```python
from build123d import *

# Parameters (mm, degrees)
F0_W      = 38
F0_H      = 28.5
F1_DEPTH  = 19.5
F2_W      = 8
F2_H      = 15.5
F4_DEPTH  = 38
F6_DEPTH  = 19.5
F3_W      = 10
F3_H      = 9
F7_DEPTH  = 38
F9_DEPTH  = 38
F11_DEPTH = 7
F12_W     = 32
F12_H     = 5
F13_DEPTH = 19
F14_R     = 2
F15_DEPTH = 4


with BuildPart() as f1:
    # F0 (on Top) → F1 (new body)
    with BuildSketch(Plane.XY):
        with Locations((3.113019, 14.25)):
            Rectangle(F0_W, F0_H)
    extrude(amount=F1_DEPTH)

    # F2 (on face) → F4 (cut)
    with BuildSketch(Plane.YZ.offset(22.113019)):
        with Locations((4, 11.75)):
            Rectangle(F2_W, F2_H)
    extrude(amount=-F4_DEPTH, mode=Mode.SUBTRACT)

    # F5 (on face) → F6 (cut)
    with BuildSketch(Plane.XY.offset(19.5)):
        with BuildLine():
            ThreePointArc((-8.449312, 27.5), (-11.386981, 18.75), (-8.449312, 10))
            Line((-8.449312, 10), (14.67535, 10))
            ThreePointArc((14.67535, 10), (17.613019, 18.75), (14.67535, 27.5))
            Line((14.67535, 27.5), (-8.449312, 27.5))
        make_face()
    extrude(amount=-F6_DEPTH, mode=Mode.SUBTRACT)

    # F3 (on face) → F7 (cut)
    with BuildSketch(Plane.YZ.offset(22.113019)):
        with Locations((23.5, 15)):
            Rectangle(F3_W, F3_H)
    extrude(amount=-F7_DEPTH, mode=Mode.SUBTRACT)

    # F8 (on face) → F9 (cut)
    with BuildSketch(Plane.YZ.offset(22.113019)):
        Polygon((18.5, 19.5), (8, 19.5), (8, 14), (10.5, 11.5), align=None)
    extrude(amount=-F9_DEPTH, mode=Mode.SUBTRACT)

    # F10 (on face) → F11 (cut)
    with BuildSketch(Plane(origin=(0, 0, 0), x_dir=(1, 0, 0), z_dir=(0, 0, -1))):
        with BuildLine():
            Line((15.550362, -9.5), (-9.324324, -9.5))
            ThreePointArc((-9.324324, -9.5), (-12.386981, -18.75), (-9.324324, -28))
            Line((-9.324324, -28), (15.550362, -28))
            ThreePointArc((15.550362, -28), (18.613019, -18.75), (15.550362, -9.5))
        make_face()
    extrude(amount=-F11_DEPTH, mode=Mode.SUBTRACT)

    # F12 (on face) → F13 (cut)
    with BuildSketch(Plane(origin=(0, 28.5, 0), x_dir=(-1, 0, 0), z_dir=(0, 1, 0))):
        with Locations((-3.113019, 2.5)):
            Rectangle(F12_W, F12_H)
    extrude(amount=-F13_DEPTH, mode=Mode.SUBTRACT)

    # F14 (on face) → F15 (cut)
    with BuildSketch(Plane.XY.offset(4)):
        with Locations((-5.136981, 4.25)):
            Circle(F14_R)
        with Locations((11.363019, 4.25)):
            Circle(F14_R)
    extrude(amount=-F15_DEPTH, mode=Mode.SUBTRACT)


solid = f1.part
```
Verification items for the finished model (mm, model axes). A direction names the side the tool comes from. Round coordinates to 2 decimals unless told otherwise and drop trailing zeros. Write each loop counter-clockwise with the first axis right and the second up, starting at its lowest first coordinate (ties: lowest second). Pieces come first, ordered by that corner, then holes. Notation, with made-up numbers: (31, -29) - (90, -29) arc R22 cw to (90, -18) - close; hole circle Ø2 at (20.5, -10). An arc over 180 degrees is marked (long way). Answer as a JSON object with one key per item and string values. Group by question number.
Q1. Tool access check on faces 1 (the flat face through (-13, 14, 15)), 2 (the flat face through (20, 18.5, 15)), 3 (the flat face through (3, 9.5, 4)). Record the directions out of +Z, -Z, +X, -X, +Y, -Y that give a thin tool (end or side, any length) a straight path to the whole face; none if there is none.
Q2. Go/stop test with flat-tipped pins: pin 1 Ø1.4 at (x, z) = (-13.5, 15) entering from +Y; pin 2 Ø1 at (x, z) = (9, 6.5) entering from -Y; pin 3 Ø4 at (x, y) = (-5, 3.5) entering from +Z; pin 4 Ø7.5 at (x, z) = (-1.5, 3.5) entering from +Y. Record where each tip stops, or that it passes through.
Q3. Section check C-C, the plane x = 7. Enter the section's corners in (y, z), plus the area to 3 significant figures.
Q4. Section check B-B, the plane z = 7.5. Enter the section's corners in (x, y), plus the area to 3 significant figures.
Q5. Mould release check, pull along Y, two halves, no side actions. Record for faces 4 (the flat face through (22.113, 17, 5)), 5 (the flat face through (-14, 18.5, 15)), 6 (the flat face through (3, 27.5, 9)): released by +Y, released by -Y, zero draft, split by the parting line, or undercut.
Q6. Section check D-D, the plane y = 14.5. Enter the section's corners in (x, z).
Q7. Section check A-A, the plane y = 4.25. Enter the section's corners in (x, z).
Q8. Thickness scan on line 1 (X direction, y = 27, z = 2); line 2 (Y direction, x = 7.5, z = 5.25); line 3 (Y direction, x = -2, z = 2.75). Record the ranges inside material, lowest first.
Found:
{
 "1": {"face 1": "+Z, +X, -X", "face 2": "+Z, +X, -X, +Y", "face 3": "-Z"},
 "2": {"pin 1": "stops at y = 18.5", "pin 2": "stops at y = 8", "pin 3": "stops at z = 4", "pin 4": "stops at y = 28.5"},
 "3": {"outline": "(0, 0) - (9.5, 0) - (9.5, 7) - (10, 7) - (10, 12) - (8, 14) - (8, 4) - (0, 4) - close; (27.5, 7) - (28, 7) - (28, 5) - (28.5, 5) - (28.5, 10.5) - (27.5, 10.5) - close", "area": "59.0 mm^2"},
 "4": {"outline": "(-15.89, 8) - (22.11, 8) - (22.11, 28.5) - (-15.89, 28.5) - close; hole (-8.45, 10) - (14.68, 10) arc R14.5 ccw to (14.68, 27.5) - (-8.45, 27.5) arc R14.5 ccw to start", "area": "304 mm^2"},
 "5": {"face 4": "zero draft", "face 5": "released by +Y", "face 6": "undercut"},
 "6": {"outline": "(-15.89, 0) - (-12.89, 0) - (-12.89, 5) - (-11.79, 5) - (-11.79, 7) - (-10.75, 7) - (-10.75, 15.5) - (-15.89, 15.5) - close; (16.98, 7) - (18.02, 7) - (18.02, 5) - (19.11, 5) - (19.11, 0) - (22.11, 0) - (22.11, 15.5) - (16.98, 15.5) - close"},
 "7": {"outline": "(-15.89, 0) - (-7.14, 0) - (-7.14, 4) - (-15.89, 4) - close; (-3.14, 0) - (9.36, 0) - (9.36, 4) - (-3.14, 4) - close; (13.36, 0) - (22.11, 0) - (22.11, 4) - (13.36, 4) - close"},
 "8": {"line 1": "x = -15.89 to -12.89, 19.11 to 22.11", "line 2": "y = 8 to 9.5, 28 to 28.5", "line 3": "y = 0 to 9.5"}
}
